The model under review builds one solid part; all positions refer to its coordinate system, in mm. Face numbers are marked on the shaded views. Coordinates: 2 decimals unless noted, no trailing zeros. Order: outer loops, then holes, each group sorted by start corner. A loop starts at its lowest first (then second) coordinate and runs counter-clockwise, first axis right, second up. Notation, with made-up numbers: M 15,-13.5 L 44,-13.5 A11 cw 44,4.5 Z; hole C 55,-39.5 d3. An arc over 180 degrees is marked long. Answer in a Markdown table with one row per item.
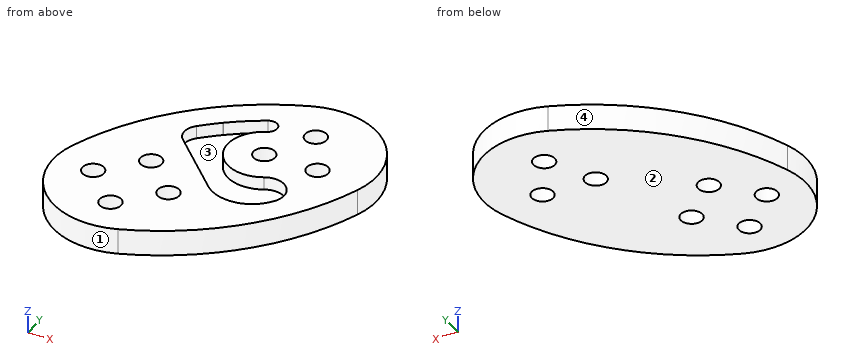
Autodesk Inventor part; units mm, degrees
ref_plane "YZ Plane" through (0, 0, 0) normal (1, 0, 0) x (0, 1, 0)
ref_plane "XZ Plane" through (0, 0, 0) normal (0, 1, 0) x (-1, 0, 0)
ref_plane "XY Plane" through (0, 0, 0) normal (0, 0, 1) x (1, 0, 0)
sketch "Sketch2" plane through (0, 0, 0) normal (0, 0, 1) x (1, 0, 0)
  line L0 (-12.7279, -12.7279) -> (0, 0) construction
  line L1 (-12.7279, -12.7279) -> (-7.4558, -12.7279) construction
  line L2 (-12.7279, -12.7279) -> (0, 0) construction
  line L3 (-17.252, -29.9799) -> (-9.2664, -21.9943) construction
  line L4 (-2.9446, 9.7833) -> (-10.9302, 1.7977) construction
  arc A0 (-21.1882, -9.6582) -> (-9.6582, -21.1882) centre (-12.7279, -12.7279) ccw
  arc A1 (8.4603, -3.0697) -> (-3.0697, 8.4603) centre (0, 0) ccw
  circle A2 centre (-8.3439, -12.7279) radius 1.25
  circle A3 centre (-8.3439, -12.7279) radius 3.1 construction
  circle A4 centre (-12.7279, -8.3439) radius 1.25
  circle A5 centre (-12.7279, -8.3439) radius 3.1 construction
  circle A6 centre (-17.112, -12.7279) radius 1.25
  circle A7 centre (-17.112, -12.7279) radius 3.1 construction
  circle A8 centre (-12.7279, -17.112) radius 1.25
  circle A9 centre (-12.7279, -17.112) radius 3.1 construction
  circle A10 centre (-3.1, -1.7898) radius 1.25
  circle A11 centre (-3.1, -1.7898) radius 3.1 construction
  circle A12 centre (3.1, -1.7898) radius 3.1 construction
  circle A13 centre (3.1, -1.7898) radius 1.25
  circle A14 centre (0, 3.5796) radius 3.1 construction
  circle A15 centre (0, 3.5796) radius 1.25
  arc A16 (-9.6582, -21.1882) -> (8.4603, -3.0697) centre (-19.9758, 7.2478) ccw
  line L5 (1.4142, -14.1421) -> (-6.364, -6.364) construction
  arc A17 (-3.0697, 8.4603) -> (-21.1882, -9.6582) centre (7.2478, -19.9758) ccw
  point P0 (-6.364, -6.364)
  dimension "d34" = 18
  dimension "d35" = 9
  dimension "d36" = 2.5
  dimension "d37" = 6.2
  dimension "d38" = 360
  dimension "d39" = 2.5
  dimension "d40" = 6.2
  dimension "d41" = 360
  dimension "d42" = 11
  dimension "d43" = 45
extrude "Extrusion2" add sketch "Sketch2" along normal blind 3
sketch "Sketch3" plane through (0, 0, 3) normal (0, 0, 1) x (1, 0, 0)
  circle A0 centre (-12.7279, -8.3439) radius 1.25
  circle A1 centre (-8.3439, -12.7279) radius 1.25
  arc A2 (-3.0697, 8.4603) -> (-21.1882, -9.6582) centre (7.2478, -19.9758) ccw
  arc A3 (-9.6582, -21.1882) -> (8.4603, -3.0697) centre (-19.9758, 7.2478) ccw
  circle A4 centre (-3.1, -1.7898) radius 1.25
  circle A5 centre (3.1, -1.7898) radius 1.25
  circle A6 centre (0, 3.5796) radius 1.25
  arc A7 (-9.6056, 1.4374) -> (-9.622, 1.4245) centre (7.2478, -19.9758) ccw
  circle A8 centre (-12.7279, -8.3439) radius 1.25
  line L0 (-11.844, -7.46) -> (-7.46, -11.844) construction
  arc A9 (1.7167, -9.2445) -> (1.8856, -9.02) centre (-19.9758, 7.2478) ccw
  line L1 (-11.7716, -3.2898) -> (-5.3387, -9.7227)
  line L2 (-5.8854, -0.7722) -> (-0.4613, -6.1962) construction
  arc A10 (1.8856, -9.02) -> (-1.1039, -5.5419) centre (0, -7.6169) ccw
  arc A11 (-5.3387, -9.7227) -> (1.7167, -9.2445) centre (-2.0197, -6.4038) ccw
  circle A12 centre (-8.3439, -12.7279) radius 4.25 construction
  circle A13 centre (-3.1, -1.7898) radius 4.25 construction
  circle A14 centre (3.1, -1.7898) radius 4.25 construction
  circle A15 centre (-12.7279, -8.3439) radius 4.25 construction
  arc A16 (-11.7519, -0.4419) -> (-11.7716, -3.2898) centre (-10.3574, -1.8755) ccw
  arc A17 (-7.1444, 3.1635) -> (-14.769, -3.9189) centre (7.2478, -19.9758) ccw construction
  arc A18 (-4.8412, 2.0872) -> (-1.1039, -5.5419) centre (-3.1, -1.7898) ccw
  arc A19 (-5.7709, 3.9632) -> (-11.7519, -0.4419) centre (7.2478, -19.9758) ccw
  arc A20 (-4.8412, 2.0872) -> (-5.7709, 3.9632) centre (-5.2704, 3.0429) ccw
  circle A21 centre (0, 3.5796) radius 4.25 construction
  point P0 (0, 0)
  point P1 (-1.1039, -5.5419)
  dimension "d46" = 3
  dimension "d49" = 3
  dimension "d52" = 3
  dimension "d53" = 3
  dimension "d54" = 3
  dimension "d55" = 3
  dimension "d56" = 3
  dimension "d59" = 3
  dimension "d60" = 2
extrude "Extrusion3" cut sketch "Sketch3" against normal blind 1.5 contours A19 A20 A18 A10 A9 A11 L1 A16 A7
sketch "sesaku" plane through (0, 0, 3) normal (0, 0, 1) x (1, 0, 0)
  arc A0 (-5.3387, -9.7227) -> (1.7167, -9.2445) centre (-2.0197, -6.4038) ccw
  line L0 (-5.3387, -9.7227) -> (-11.7716, -3.2898)
  arc A1 (-11.7519, -0.4419) -> (-11.7716, -3.2898) centre (-10.3574, -1.8755) ccw
  arc A2 (1.8856, -9.02) -> (-1.1039, -5.5419) centre (0, -7.6169) ccw
  arc A3 (1.7167, -9.2445) -> (1.8856, -9.02) centre (-19.9758, 7.2478) ccw
  arc A4 (-9.6582, -21.1882) -> (8.4603, -3.0697) centre (-19.9758, 7.2478) ccw
  arc A5 (8.4603, -3.0697) -> (-3.0697, 8.4603) centre (0, 0) ccw
  arc A6 (-3.0697, 8.4603) -> (-21.1882, -9.6582) centre (7.2478, -19.9758) ccw
  arc A7 (-21.1882, -9.6582) -> (-9.6582, -21.1882) centre (-12.7279, -12.7279) ccw
  circle A8 centre (0, 3.5796) radius 1.25
  circle A9 centre (3.1, -1.7898) radius 1.25
  circle A10 centre (-3.1, -1.7898) radius 1.25
  circle A11 centre (-12.7279, -17.112) radius 1.25
  circle A12 centre (-17.112, -12.7279) radius 1.25
  circle A13 centre (-12.7279, -8.3439) radius 1.25
  circle A14 centre (-8.3439, -12.7279) radius 1.25
  arc A15 (-5.7709, 3.9632) -> (-11.7519, -0.4419) centre (7.2478, -19.9758) ccw
  arc A16 (-4.8412, 2.0872) -> (-5.7709, 3.9632) centre (-5.2704, 3.0429) ccw
  arc A17 (-4.8412, 2.0872) -> (-1.1039, -5.5419) centre (-3.1, -1.7898) ccw
properties part number "駆動節" material "Aluminum 2014-T6"
(1) Insertion check: P1, Ø2, axis at x = -12.73, y = -17.11, coming from the +Z side; P2, Ø1, axis at x = 3, z = 2.5, coming from the -Y side; P3, Ø1.5, axis at y = -8, z = 2.5, coming from the +X side. Each pin has a flat end and moves straight along its axis. Give the tip position at first contact, or say it passes through.
Report:
| item | result |
|---|---|
| P1 | through |
| P2 | y = -13 |
| P3 | x = 6.57 |
(2) Take a section at C-C (z = 2.3). State how many separate pieces and enclosed holes the cut face has, then the cut area to 3 significant figures.
Report:
| item | result |
|---|---|
| separate pieces | 1 |
| enclosed holes | 8 |
| area | 519 mm^2 |
(3) To check wall thickness, follow line 1 (X direction, y = -13, z = 0.2); line 2 (X direction, y = -2.5, z = 0.45); line 3 (Z direction, x = 1, y = -9.5). State the ranges of each line that lie inside material, in increasing order. Write a range as [from, to].
Report:
| item | result |
|---|---|
| line 1 | [-21.72, -18.33], [-15.89, -9.56], [-7.12, 2.5] |
| line 2 | [-17.44, -4.13], [-2.07, 2.07], [4.13, 8.65] |
| line 3 | [0, 1.5] |
(4) Take a section at B-B (y = 0.5). Write out the cut boundary in (x, z), then the cut area to 3 significant figures.
Report:
| item | result |
|---|---|
| outline | M -15.02,0 L 8.99,0 L 8.99,3 L -6.68,3 L -6.68,1.5 L -10.73,1.5 L -10.73,3 L -15.02,3 Z |
| area | 65.9 mm^2 |
(5) Take a section at A-A (x = -2.5). Write out the cut boundary in (y, z), then the cut area to 3 significant figures.
Report:
| item | result |
|---|---|
| outline | M -17.44,0 L -2.89,0 L -2.89,3 L -6,3 L -6,1.5 L -11.07,1.5 L -11.07,3 L -17.44,3 Z; M -0.69,0 L 8.65,0 L 8.65,3 L -0.69,3 Z |
| area | 64.1 mm^2 |
(6) The part is to be moulded in two halves that separate along X. For the marked faces 1, 2, 3 and 4, say which applies: +X half, -X half, draft (parallel to the pull), parting line (faces both ways), or undercut.
Report:
| item | result |
|---|---|
| face 1 | parting line |
| face 2 | draft |
| face 3 | undercut |
| face 4 | -X half |
(7) Take a section at D-D (x = 3.1). Write out the cut boundary in (y, z), then the cut area to 3 significant figures.
Report:
| item | result |
|---|---|
| outline | M -12.31,0 L -3.04,0 L -3.04,3 L -12.31,3 Z; M -0.54,0 L 8.45,0 L 8.45,3 L -0.54,3 Z |
| area | 54.8 mm^2 |
